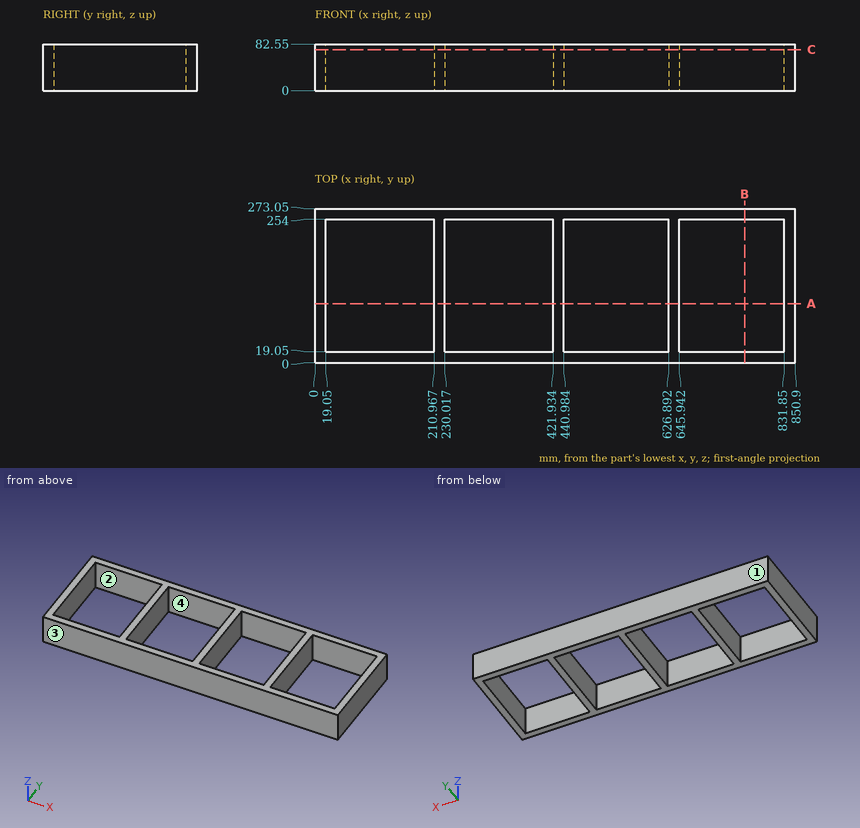
Here's the drawing with two shaded views (mm, measured from the low corner). I have some questions. A direction names the side the tool comes from. Coordinates: 2 decimals unless noted, no trailing zeros. Write each loop counter-clockwise with the first axis right and the second up, starting at its lowest first coordinate (ties: lowest second). Pieces come first, ordered by that corner, then holes.
Item 1: Will this pin go through, and if not, where does the flat tip stop? pin 1 (3 mm diameter, centred on y = 95.5, z = 67.5, fed in from -X).
Item 2: I want a section at B-B on x = 761.5. Write out the boundary of the cut face in (y, z), and give its area (3 significant figures).
Item 3: I want a section at A-A on y = 104.5. Write out the boundary of the cut face in (x, z).
Item 4: On a 3-axis mill with a long thin cutter (end or side, diameter ignored), from which of +Z, -Z, +X, -X, +Y, -Y can I reach the whole of each face in a straight line? I mean the marked faces 3 and 4. Say none if no direction works.
Item 5: If I drill on line 1 (X direction, y = 145, z = 62); line 2 (Y direction, x = 332, z = 26), over which ranges is the centre line in solid material (lowest first)?
Item 6: If we mould it in two halves opening along X, with no side actions, what happens to the marked faces 1 and 2? For each: +X half, -X half, draft (parallel to the pull), parting line (faces both ways), or undercut.
Item 7: I want a section at C-C on z = 72.5. Write out the boundary of the cut face in (x, y).
Findings below:
1. pin 1: stops at x = 0
2. outline: (0, 0) - (19.05, 0) - (19.05, 82.55) - (0, 82.55) - close; (254, 0) - (273.05, 0) - (273.05, 82.55) - (254, 82.55) - close
2. area: 3,150 mm2
3. outline: (0, 0) - (19.05, 0) - (19.05, 82.55) - (0, 82.55) - close; (210.97, 0) - (230.02, 0) - (230.02, 82.55) - (210.97, 82.55) - close; (421.93, 0) - (440.98, 0) - (440.98, 82.55) - (421.93, 82.55) - close; (626.89, 0) - (645.94, 0) - (645.94, 82.55) - (626.89, 82.55) - close; (831.85, 0) - (850.9, 0) - (850.9, 82.55) - (831.85, 82.55) - close
4. face 3: +Z, -Z, +X, -X, -Y
4. face 4: +Z, -Z
5. line 1: x = 0 to 19.05, 210.97 to 230.02, 421.93 to 440.98, 626.89 to 645.94, 831.85 to 850.9
5. line 2: y = 0 to 19.05, 254 to 273.05
6. face 1: draft
6. face 2: undercut
7. outline: (0, 0) - (850.9, 0) - (850.9, 273.05) - (0, 273.05) - close; hole (19.05, 19.05) - (210.97, 19.05) - (210.97, 254) - (19.05, 254) - close; hole (230.02, 19.05) - (421.93, 19.05) - (421.93, 254) - (230.02, 254) - close; hole (440.98, 19.05) - (626.89, 19.05) - (626.89, 254) - (440.98, 254) - close; hole (645.94, 19.05) - (831.85, 19.05) - (831.85, 254) - (645.94, 254) - close
